```python
from build123d import *

# Parameters (mm, degrees)
EXTRUDE_THIN1_DEPTH = 76.2
EXTRUDE1_REACH      = 107.917
EXTRUDE1_END_RADIUS = 76.967998962
SKETCH2_R           = 22.797803907
SKETCH3_R           = 18.98465739
EXTRUDE2_DEPTH      = 76.2


with BuildPart() as part:
    # Sketch1 → Extrude-Thin1 (new body)
    with BuildSketch(Plane(origin=(0, 0, 0), x_dir=(0, 0, -1), z_dir=(1, 0, 0))):
        with BuildLine():
            ThreePointArc((-40.374745946, 0), (12.536707256, 21.071210286), (65.448160458, 0))
            Line((65.448160458, 0), (63.702043982, -1.84463472))
            ThreePointArc((63.702043982, -1.84463472), (12.536707256, 18.531210286), (-38.628629469, -1.84463472))
            Line((-38.628629469, -1.84463472), (-40.374745946, 0))
        make_face()
    extrude(amount=-EXTRUDE_THIN1_DEPTH)

    # Extrude1: up to this cylinder (the profile starts outside it)
    extrude1_end = Plane(origin=(-37.931127, -55.896788676, -12.536707256), z_dir=(1, 0, 0)) * Cylinder(EXTRUDE1_END_RADIUS, 370.769997925, mode=Mode.PRIVATE)
    # Sketch2 → Extrude1 (add, up to the surface)
    with BuildSketch(Plane(origin=(0, 31.75, 0), x_dir=(-1, 0, 0), z_dir=(0, 1, 0)), mode=Mode.PRIVATE) as extrude1_sk1:
        with Locations(Location((37.931127378, -9.159254826, 0), (0, 0, 90))):
            Circle(SKETCH2_R)
    extrude1_tool1 = extrude(extrude1_sk1.sketch, amount=-EXTRUDE1_REACH, mode=Mode.PRIVATE) - extrude1_end
    add(extrude1_tool1.solids().sort_by_distance((-37.931127, 31.75, -9.159255))[0])

    # Sketch3 → Extrude2 (cut)
    with BuildSketch(Plane(origin=(0, 31.75, 0), x_dir=(-1, 0, 0), z_dir=(0, 1, 0))):
        with Locations(Location((37.931127378, -9.159254826, 0), (0, 0, 90))):
            Circle(SKETCH3_R)
    extrude(amount=-EXTRUDE2_DEPTH, mode=Mode.SUBTRACT)


solid = part.part
```
The listing builds one solid part. Answer for the finished solid, in the listing's coordinates (mm). A direction names the side the tool comes from. Round coordinates to 2 decimals unless told otherwise and drop trailing zeros. Loops run counter-clockwise (first coordinate to the right, second up) from the corner with the lowest first, then second, coordinate; pieces in that order, holes last.
1) Consider line 1 (Z direction, x = -44.5, y = 23.5); line 2 (Z direction, x = -26, y = 20); line 3 (X direction, y = 27.5, z = 5). Determine where each line is inside the solid, lowest interval first.
Outcome:
line 1: z = -30.99 to -26.97, 8.65 to 12.67
line 2: z = -28.59 to -23.93, 5.61 to 10.27
line 3: x = -55.8 to -50.58, -25.28 to -20.06
2) A cutting plane is placed at D-D on x = -64. Determine the outline of the cut face in (y, z).
Outcome:
outline: (-1.84, -63.7) - (0, -65.45) arc R76.97 ccw to (0, 40.37) - (-1.84, 38.63) arc R74.43 cw to start
3) A cutting plane is placed at A-A on y = 4.5. Determine the outline of the cut face in (x, z).
Outcome:
outline: (-76.2, -60.25) - (0, -60.25) - (0, -56.03) - (-76.2, -56.03) - close; (-76.2, 30.96) - (0, 30.96) - (0, 35.17) - (-76.2, 35.17) - close
4) A cutting plane is placed at B-B on z = -22.5. Determine the outline of the cut face in (x, y), plus the area to 3 significant figures.
Outcome:
outline: (-76.2, 17.86) - (-51.44, 17.86) - (-51.44, 31.75) - (-56.42, 31.75) - (-56.42, 20.42) - (-76.2, 20.42) - close; (-24.42, 17.86) - (0, 17.86) - (0, 20.42) - (-19.44, 20.42) - (-19.44, 31.75) - (-24.42, 31.75) - close
area: 239 mm2
5) A cutting plane is placed at C-C on x = -21.5. Determine the outline of the cut face in (y, z).
Outcome:
outline: (-1.84, -63.7) - (0, -65.45) arc R76.97 ccw to (20.06, -24.96) - (31.75, -24.96) - (31.75, -18.67) - (18.28, -18.67) arc R74.43 cw to start; (-1.84, 38.63) arc R74.43 cw to (17.41, 0.35) - (31.75, 0.35) - (31.75, 6.64) - (18.64, 6.64) arc R76.97 ccw to (0, 40.37) - close
6) For faces 1 (the face through (-19, 31.75, -14)), 2 (the face through (-31.083, 25.92, 12.586)), determine the directions among +Z, -Z, +X, -X, +Y, -Y from which every point of the face is accessible in a straight line to the end or side of a thin tool.
Outcome:
face 1: +Z, -Z, +X, -X, +Y
face 2: +Y
7) Given P1, Ø3, axis at x = -64, z = 4, coming from the -Y side; P2, Ø4, axis at x = -66.5, z = 25, coming from the +Y side; P3, Ø12, axis at x = -42, y = 14, coming from the +Z side, each flat-ended and moving along its own axis, determine where each tip first touches the part or whether it passes through.
Outcome:
P1: stops at y = 16.31
P2: stops at y = 12.38
P3: stops at z = 30.37
